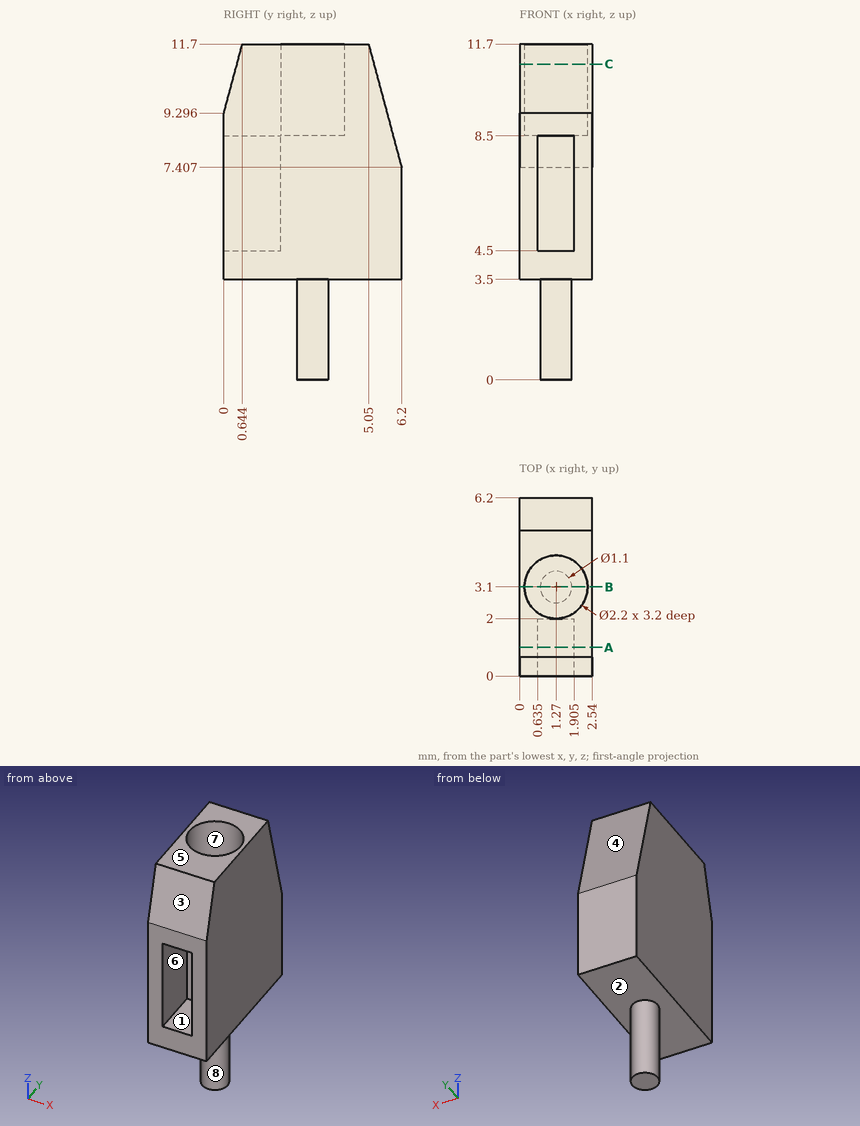
For this review, use the dimensioned drawing (mm, ordinates from the lowest corner) and the shaded views. A direction names the side the tool comes from. Coordinates: 2 decimals unless noted, no trailing zeros. Loops run counter-clockwise (first coordinate to the right, second up) from the corner with the lowest first, then second, coordinate; pieces in that order, holes last.
1. For the marked faces 4, 5, 6, 7 and 8, list the 3-axis set-ups (+Z, -Z, +X, -X, +Y, -Y) from which the entire face can be reached by the end or side of a thin tool; tool diameter is ignored.
2. Mouldability with a two-part tool opening along Z and no side actions: class the marked faces 1, 2 and 3 as +Z half, -Z half, draft (parallel to the pull), parting line (faces both ways), or undercut.
3. For line 1 (X direction, y = 3.1, z = 9.9); line 2 (Z direction, x = 1.25, y = 1); line 3 (Y direction, x = 1.1, z = 5.5), list the stretches that pass through material, from the lowest coordinate up.
4. Add section C-C, the plane z = 11. Give the boundary of the cut face in (x, y).
5. Insertion check: P1, Ø0.7, axis at x = 1, y = 3, coming from the +Z side; P2, Ø1.4, axis at x = 1, y = 0.5, coming from the -Z side. Each pin has a flat end and moves straight along its axis. Give the tip position at first contact, or say it passes through.
6. Add section B-B, the plane y = 3.1. Give the boundary of the cut face in (x, z).
7. Add section A-A, the plane y = 1. Give the boundary of the cut face in (x, z) (1 decimal).
Result:
1. face 4: +Z, +X, -X, +Y
1. face 5: +Z, +X, -X, +Y, -Y
1. face 6: -Y
1. face 7: +Z
1. face 8: -Z
2. face 1: undercut
2. face 2: -Z half
2. face 3: +Z half
3. line 1: x = 0 to 0.17, 2.37 to 2.54
3. line 2: z = 3.5 to 4.5, 8.5 to 11.7
3. line 3: y = 2 to 6.2
4. outline: (0, 0.46) - (2.54, 0.46) - (2.54, 5.24) - (0, 5.24) - close; hole circle Ø2.2 at (1.27, 3.1)
5. P1: stops at z = 8.5
5. P2: stops at z = 3.5
6. outline: (0, 3.5) - (0.72, 3.5) - (0.72, 0) - (1.82, 0) - (1.82, 3.5) - (2.54, 3.5) - (2.54, 11.7) - (2.37, 11.7) - (2.37, 8.5) - (0.17, 8.5) - (0.17, 11.7) - (0, 11.7) - close
7. outline: (0, 3.5) - (2.5, 3.5) - (2.5, 11.7) - (0, 11.7) - close; hole (0.6, 4.5) - (1.9, 4.5) - (1.9, 8.5) - (0.6, 8.5) - close
